For this review, take the finished solid that the model builds, in its own axes (mm). A direction names the side the tool comes from. Coordinates: 2 decimals unless noted, no trailing zeros. Order: outer loops, then holes, each group sorted by start corner. A loop starts at its lowest first (then second) coordinate and runs counter-clockwise, first axis right, second up. Notation, with made-up numbers: (42, 77) -> (68, 77) arc R13 ccw to (68, 98) -> close; hole circle Ø7 at (68.25, 3). An arc over 180 degrees is marked (long way). Answer as a JSON object with one key per item and string values. Group by question number.
1) For pin 1 (10 mm diameter, centred on x = 5.5, y = 53.5, fed in from -Z); pin 2 (4 mm diameter, centred on x = -12.5, z = 7, fed in from -Y); pin 3 (4 mm diameter, centred on y = 127, z = -5, fed in from +X); pin 4 (7.5 mm diameter, centred on x = 0, z = 0, fed in from +Y), all flat-tipped, find the tip position at first contact; note any pin that passes through.
2) Add section A-A, the plane z = 0. Write out the cut boundary in (x, y), then the cut area to 3 significant figures.
3) Draft analysis for pull direction Z (two halves, no side actions). For faces 3 (the cylindrical face through (-1.38, 111.2, -6.2)), 4 (the flat face through (-25.4, 4, 0)), 5 (the cylindrical face through (-3.597, 120.965, -16.196)), state which applies: +Z half, -Z half, draft (parallel to the pull), parting line (faces both ways), or undercut.
4) Machinability: for faces 1 (the flat face through (5, 0, 6)), 2 (the flat face through (10, 11.176, 16)), which of the approach directions +Z, -Z, +X, -X, +Y, -Y give a long, thin tool a straight path to every point of the face, cutting with its end or side? Answer none if there is none.
5) Add section B-B, the plane x = 0. Write out the cut boundary in (y, z), then the cut area to 3 significant figures.
6) Add section D-D, the plane z = 20.5. Write out the cut boundary in (x, y).
7) Wall thickness on L1, parallel to Z at x = 0, y = 71; L2, parallel to Y at x = 23, z = 3.5; L3, parallel to Z at x = -1.5, y = 54.5: over which ranges is each line inside the solid? List them lowest first.
8) Add section C-C, the plane y = 21. Write out the cut boundary in (x, z), then the cut area to 3 significant figures.
from build123d import *

# Parameters (mm, degrees)
F0_W     = 50.8
F0_H     = 50.8
F0_R     = 16.5908146865
F1_DEPTH = 11.176
F0_R_2   = 6.35
F2_DEPTH = 235.712
F3_R     = 2.4528409794
F4_R     = 2.4528409794
F5_R     = 2.4528409794
F6_R     = 2.4528409794
F7_R     = 1.8396307345


# Not quite as in the source:
# - a fillet or chamfer that OpenCascade refuses, or shapes differently, is made with other operations: its cross-section is extruded or revolved along the edge and cut away or added


with BuildPart() as f1:
    # F0 (on Front) → F1 (new body)
    with BuildSketch(Plane.XZ):
        Rectangle(F0_W, F0_H)
        Circle(F0_R, mode=Mode.SUBTRACT)
    extrude(amount=-F1_DEPTH)

    # F0 (on Front) → F2 (join)
    with BuildSketch(Plane.XZ):
        Circle(F0_R)
        Circle(F0_R_2, mode=Mode.SUBTRACT)
    extrude(amount=-F2_DEPTH)

    # F3
    f3_edges = [f1.edges().sort_by_distance(p)[0] for p in [
        (-25.4, 11.176, 0),
    ]]
    fillet(f3_edges, radius=F3_R)

    # F4
    f4_edges = [f1.edges().sort_by_distance(p)[0] for p in [
        (1.22642, 11.176, 25.4),
    ]]
    fillet(f4_edges, radius=F4_R)

    # F5
    f5_edges = [f1.edges().sort_by_distance(p)[0] for p in [
        (25.4, 11.176, -1.22642),
    ]]
    fillet(f5_edges, radius=F5_R)

    # F6
    f6_edges = [f1.edges().sort_by_distance(p)[0] for p in [
        (0, 11.176, -25.4),
    ]]
    fillet(f6_edges, radius=F6_R)

    # F7
    f7_edges = [f1.edges().sort_by_distance(p)[0] for p in [
        (-16.590815, 235.712, 0),
    ]]
    fillet(f7_edges, radius=F7_R)

    # F8: chamfer of 10.16 on 1 edges, made by hand

    # F8_s1 → F8_t2 (revolve, cut)
    with BuildSketch(Plane.XY):
        Polygon((16.51, 235.712), (6.35, 225.552), (6.35, 235.712), align=None)
    revolve(axis=Axis((0, 235.712, 0), (0, -1, 0)), mode=Mode.SUBTRACT)


solid = f1.part
Output values:
{
 "1": {"pin 1": "stops at z = -16.58", "pin 2": "stops at y = 0", "pin 3": "stops at x = 16.32", "pin 4": "passes through"},
 "2": {"outline": "(-25.4, 0) -> (-6.35, 0) -> (-6.35, 225.55) -> (-16.01, 235.21) arc R1.84 ccw to (-16.59, 233.87) -> (-16.59, 11.18) -> (-22.95, 11.18) arc R2.45 ccw to (-25.4, 8.72) -> close; (6.35, 0) -> (25.4, 0) -> (25.4, 8.72) arc R2.45 ccw to (22.95, 11.18) -> (16.59, 11.18) -> (16.59, 233.87) arc R1.84 ccw to (16.01, 235.21) -> (6.35, 225.55) -> close", "area": "4,920 mm²"},
 "3": {"face 3": "undercut", "face 4": "draft", "face 5": "parting line"},
 "4": {"face 1": "+Z, -Z, +X, -X, -Y", "face 2": "+Y"},
 "5": {"outline": "(0, -25.4) -> (8.72, -25.4) arc R2.45 ccw to (11.18, -22.95) -> (11.18, -16.59) -> (233.87, -16.59) arc R1.84 ccw to (235.21, -16.01) -> (225.55, -6.35) -> (0, -6.35) -> close; (0, 6.35) -> (225.55, 6.35) -> (235.21, 16.01) arc R1.84 ccw to (233.87, 16.59) -> (11.18, 16.59) -> (11.18, 22.95) arc R2.45 ccw to (8.72, 25.4) -> (0, 25.4) -> close", "area": "4,920 mm²"},
 "6": {"outline": "(-25.4, 0) -> (25.4, 0) -> (25.4, 8.72) arc R2.45 ccw to (22.95, 11.18) -> (-22.95, 11.18) arc R2.45 ccw to (-25.4, 8.72) -> close"},
 "7": {"L1": "z = -16.59 to -6.35, 6.35 to 16.59", "L2": "y = 0 to 11.18", "L3": "z = -16.52 to -6.17, 6.17 to 16.52"},
 "8": {"outline": "circle Ø33.18 at (0, 0); hole circle Ø12.7 at (0, 0)", "area": "738 mm²"}
}
